Model file for the job. Use its own axes, mm. Give positions to 0.01 mm unless a question says otherwise; leave off trailing zeros. Write each loop counter-clockwise with the first axis right and the second up, starting at its lowest first coordinate (ties: lowest second). Pieces come first, ordered by that corner, then holes. Notation, with made-up numbers: (18.25, 81) - (35.25, 81) arc R28 ccw to (35.25, 118) - close; hole circle Ø5 at (88, 7). An arc over 180 degrees is marked (long way). Use a Markdown table: item, result. Add a question column.
Autodesk Inventor part; units mm, degrees
ref_plane "YZ Plane" through (0, 0, 0) normal (1, 0, 0) x (0, 1, 0)
ref_plane "XZ Plane" through (0, 0, 0) normal (0, 1, 0) x (-1, 0, 0)
ref_plane "XY Plane" through (0, 0, 0) normal (0, 0, 1) x (1, 0, 0)
sketch "Boceto1" plane through (0, 0, 0) normal (0, 1, 0) x (-1, 0, 0)
  line L0 (41.5, 18) -> (-41.5, 18)
  line L1 (-41.5, 18) -> (-41.5, -18)
  line L2 (-41.5, -18) -> (41.5, -18)
  line L3 (41.5, -18) -> (41.5, 18)
  line L4 (41.5, 18) -> (-41.5, -18) construction
  line L5 (-41.5, 18) -> (41.5, -18) construction
  point P0 (0, 0)
  dimension "d0" = 83
  dimension "d1" = 36
extrude "Extrusión1" add sketch "Boceto1" along normal blind 1
sketch "Boceto2" plane through (0, 1, 0) normal (0, 1, 0) x (1, 0, 0)
  line L0 (41.5, 18) -> (-41.5, 18)
  line L1 (-41.5, 18) -> (-18.7131, 18) construction
  circle A0 centre (-39.5, 16) radius 1
  circle A1 centre (39.5, 13) radius 1
  circle A2 centre (-39.5, -13) radius 1
  circle A3 centre (39.5, -13) radius 1
  point P0 (0, 0)
  dimension "d5" = 2
  dimension "d6" = 2
extrude "Extrusión2" cut sketch "Boceto2" against normal through all
properties part number "PCB"
(1) Band-saw the part on A-A (z = -13). Write the cut outline in (x, y).
(2) Band-saw the part on C-C (x = -39.5). Write the cut outline in (y, z).
(3) Band-saw the part on B-B (z = 13). Write the cut outline in (x, y), then the cut area to 3 significant figures.
(4) Probe probe 1 along X at (y, z) = (0.5, 13); probe 2 along Z at (x, y) = (-39.5, 0.5); probe 3 along Z at (x, y) = (39.5, 0.7). List the from-to ranges inside material, lowest first. Write a range as [from, to].
(5) Two-plate mould, pull along Z, no slides. Class faces 1 (the flat face through (1, 0, 0)), 2 (the cylindrical face through (40.424, 0.507, 13.383)): +Z half, -Z half, draft (parallel to the pull), parting line (faces both ways), or undercut.
(6) Flat gauge pins, fed straight in: pin 1 (8 mm diameter, centred on x = -18, z = -12.5, fed in from -Y); pin 2 (1.2 mm diameter, centred on x = -39.5, z = 13, fed in from -Y). Where does each tip first touch, or does it go through?
Model answer:
| question | item | result |
|---|---|---|
| 1 | outline | (-41.5, 0) - (38.5, 0) - (38.5, 1) - (-41.5, 1) - close; (40.5, 0) - (41.5, 0) - (41.5, 1) - (40.5, 1) - close |
| 2 | outline | (0, -18) - (1, -18) - (1, -17) - (0, -17) - close; (0, -15) - (1, -15) - (1, 12) - (0, 12) - close; (0, 14) - (1, 14) - (1, 18) - (0, 18) - close |
| 3 | outline | (-41.5, 0) - (-40.5, 0) - (-40.5, 1) - (-41.5, 1) - close; (-38.5, 0) - (38.5, 0) - (38.5, 1) - (-38.5, 1) - close; (40.5, 0) - (41.5, 0) - (41.5, 1) - (40.5, 1) - close |
| 3 | area | 79.0 mm^2 |
| 4 | probe 1 | x = [-41.5, -40.5], [-38.5, 38.5], [40.5, 41.5] |
| 4 | probe 2 | z = [-18, -17], [-15, 12], [14, 18] |
| 4 | probe 3 | z = [-18, -14], [-12, 12], [14, 18] |
| 5 | face 1 | draft |
| 5 | face 2 | undercut |
| 6 | pin 1 | stops at y = 0 |
| 6 | pin 2 | passes through |
